```python
from build123d import *

# Parameters (mm, degrees)
F0_R            = 60
F0_R_2          = 36
F1_DEPTH        = 2
F2_R            = 5
F3_DEPTH        = 2.001
F3_COPIES_COUNT = 6


# Not quite as in the source:
# - a pattern or mirror of a feature is missing from the dataset's text; its kind, count and spacing are read off the source's solid


with BuildPart() as f1:
    # F0 (on Front) → F1 (new body)
    with BuildSketch(Plane.XZ):
        Circle(F0_R)
        Circle(F0_R_2, mode=Mode.SUBTRACT)
    extrude(amount=F1_DEPTH)

    # F2 (on face) → F3 (cut, through all)
    with BuildSketch(Plane.XZ.offset(2)):
        with Locations((0, 50.5)):
            Circle(F2_R)
    f3 = extrude(amount=-F3_DEPTH, mode=Mode.SUBTRACT)

    # F3_copies: F3 ×6 about axis
    f3_copies_axis = Axis((0, 0, 0), (0, 1, 0))
    for i in range(1, F3_COPIES_COUNT):
        add(f3.rotate(f3_copies_axis, i * 360 / F3_COPIES_COUNT), mode=Mode.SUBTRACT)


solid = f1.part
```
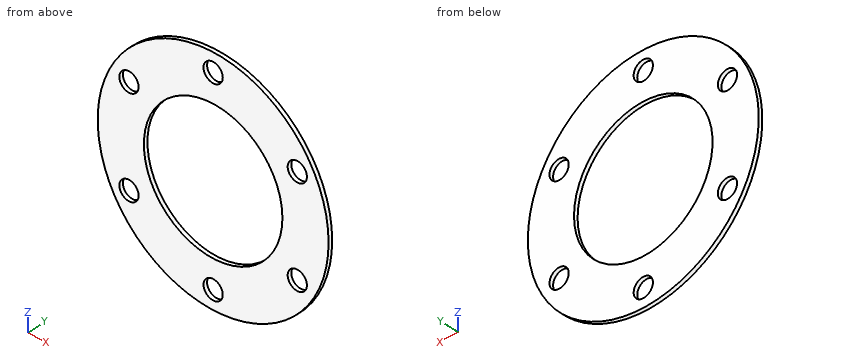
Check sheet for the modelled part. Datum: model origin and axes. Units: mm. Round coordinates to 2 decimals unless told otherwise and drop trailing zeros. Loops run counter-clockwise (first coordinate to the right, second up) from the corner with the lowest first, then second, coordinate; pieces in that order, holes last. Notation, with made-up numbers: (-38, -7) -> (-25, -7) arc R22 cw to (-25, 2) -> close; hole circle Ø7 at (62, -31). An arc over 180 degrees is marked (long way). Answer in a Markdown table with one row per item.
Q1. Sectioned sample at B-B on z = -33. Enter the section's corners in (x, y), then the cut area to 3 significant figures.
Data:
| item | result |
|---|---|
| outline | (-50.11, -2) -> (-14.39, -2) -> (-14.39, 0) -> (-50.11, 0) -> close; (14.39, -2) -> (50.11, -2) -> (50.11, 0) -> (14.39, 0) -> close |
| area | 143 mm^2 |
Q2. Go/stop test with a flat-tipped pin: P1, Ø16, axis at x = 0, z = -50.5, coming from the -Y side. Record where the tip stops, or that it passes through.
Data:
| item | result |
|---|---|
| P1 | stops at y = -2 |
Q3. Sectioned sample at C-C on x = 25.5. Enter the section's corners in (y, z), then the cut area to 3 significant figures.
Data:
| item | result |
|---|---|
| outline | (-2, -54.31) -> (0, -54.31) -> (0, -25.41) -> (-2, -25.41) -> close; (-2, 25.41) -> (0, 25.41) -> (0, 54.31) -> (-2, 54.31) -> close |
| area | 116 mm^2 |
Q4. Sectioned sample at D-D on y = -0.8. Enter the section's corners in (x, z).
Data:
| item | result |
|---|---|
| outline | circle Ø120 at (0, 0); hole circle Ø10 at (-43.73, -25.25); hole circle Ø10 at (-43.73, 25.25); hole circle Ø72 at (0, 0); hole circle Ø10 at (0, -50.5); hole circle Ø10 at (0, 50.5); hole circle Ø10 at (43.73, -25.25); hole circle Ø10 at (43.73, 25.25) |
Q5. Sectioned sample at A-A on x = 0. Enter the section's corners in (y, z).
Data:
| item | result |
|---|---|
| outline | (-2, -60) -> (0, -60) -> (0, -55.5) -> (-2, -55.5) -> close; (-2, -45.5) -> (0, -45.5) -> (0, -36) -> (-2, -36) -> close; (-2, 36) -> (0, 36) -> (0, 45.5) -> (-2, 45.5) -> close; (-2, 55.5) -> (0, 55.5) -> (0, 60) -> (-2, 60) -> close |
Q6. Thickness scan on L1, parallel to Z at x = 0, y = -0.75; L2, parallel to Z at x = 43, y = -0.35; L3, parallel to X at y = -0.4, z = 22. Record the ranges inside material, lowest first.
Data:
| item | result |
|---|---|
| L1 | z = -60 to -55.5, -45.5 to -36, 36 to 45.5, 55.5 to 60 |
| L2 | z = -41.84 to -30.2, -20.3 to 20.3, 30.2 to 41.84 |
| L3 | x = -55.82 to -47.53, -39.93 to -28.5, 28.5 to 39.93, 47.53 to 55.82 |
